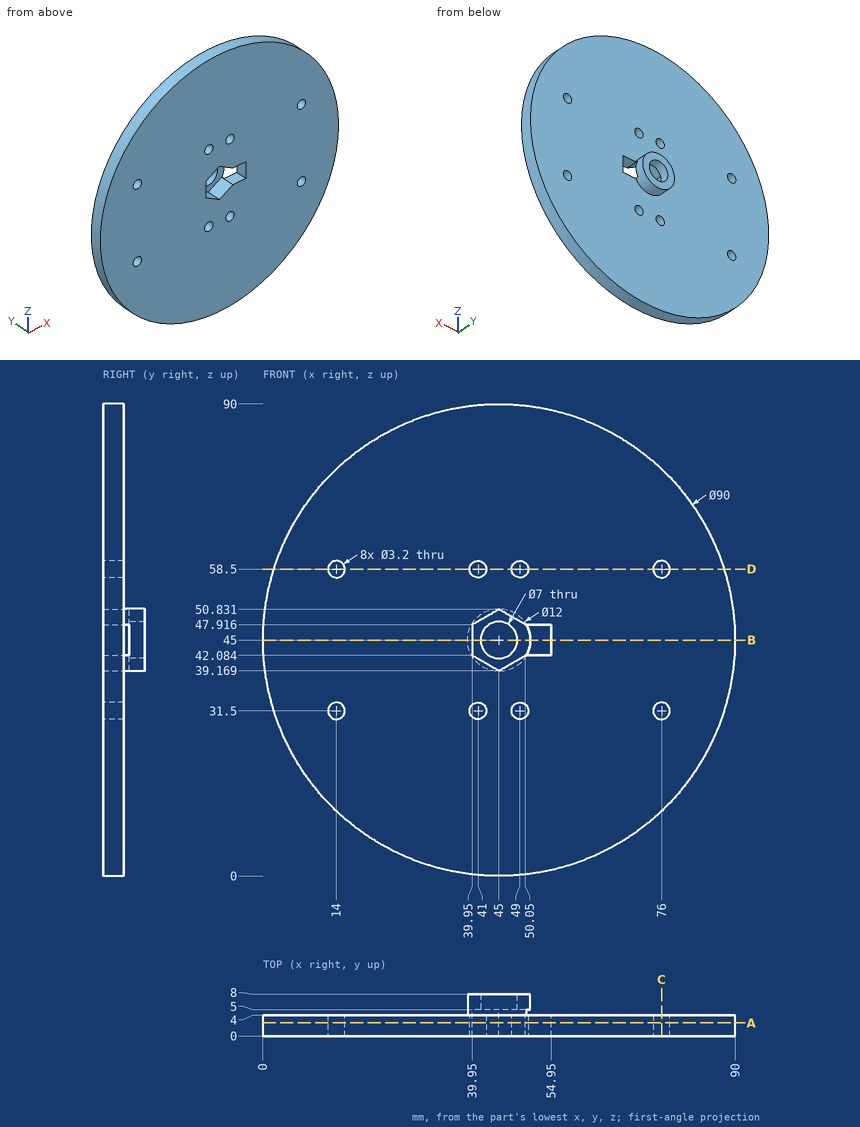
Geometry check sheet. Reference: drawing and pictorial views, mm from the part's lowest x, y, z. Round coordinates to 2 decimals unless told otherwise and drop trailing zeros. Order: outer loops, then holes, each group sorted by start corner. A loop starts at its lowest first (then second) coordinate and runs counter-clockwise, first axis right, second up. Notation, with made-up numbers: M -35.5,-8 L 6.5,-8 A28 ccw 6.5,10 Z; hole C 85.5,85 d6. An arc over 180 degrees is marked long. Answer in a Markdown table with one row per item.
(1) Scan lines: probe 1 along Z at (x, y) = (14, 1.9); probe 2 along Z at (x, y) = (49, 2.75); probe 3 along Y at (x, z) = (20, 13). Record each from-to range of solid material in increasing order. Write a range as from..to.
Responses:
| item | result |
|---|---|
| probe 1 | z = 12.38..29.9, 33.1..56.9, 60.1..77.62 |
| probe 2 | z = 0.18..29.9, 33.1..41.48, 48.52..56.9, 60.1..89.82 |
| probe 3 | y = 0..4 |
(2) Sectioned sample at C-C, the plane x = 76. Record the cut outline in (y, z), and give its area (3 significant figures).
Responses:
| item | result |
|---|---|
| outline | M 0,12.38 L 4,12.38 L 4,29.9 L 0,29.9 Z; M 0,33.1 L 4,33.1 L 4,56.9 L 0,56.9 Z; M 0,60.1 L 4,60.1 L 4,77.62 L 0,77.62 Z |
| area | 235 mm² |
(3) Sectioned sample at A-A, the plane y = 2.5. State how many separate pieces and enclosed holes the cut face has, and give its area (3 significant figures).
Responses:
| item | result |
|---|---|
| separate pieces | 1 |
| enclosed holes | 9 |
| area | 6,180 mm² |
(4) Go/stop test with flat-tipped pins: P1, Ø3, axis at x = 49, z = 58.5, coming from the -Y side; P2, Ø2.5, axis at y = 1.5, z = 43.5, coming from the +X side; P3, Ø3.5, axis at x = 76, z = 58.5, coming from the +Y side; P4, Ø2.5, axis at x = 53, y = 1.5, coming from the +Z side. Record where each tip stops, or that it passes through.
Responses:
| item | result |
|---|---|
| P1 | passes through |
| P2 | stops at x = 90 |
| P3 | stops at y = 4 |
| P4 | stops at z = 89.49 |
(5) Sectioned sample at B-B, the plane z = 45. Record the cut outline in (x, y), and give its area (3 significant figures).
Responses:
| item | result |
|---|---|
| outline | M 0,0 L 39.95,0 L 39.95,5 L 41.5,5 L 41.5,8 L 39,8 L 39,4 L 0,4 Z; M 48.5,5 L 51,5 L 51,8 L 48.5,8 Z; M 54.95,0 L 90,0 L 90,4 L 54.95,4 Z |
| area | 316 mm² |
(6) Sectioned sample at D-D, the plane z = 58.5. Record the cut outline in (x, y), and give its area (3 significant figures).
Responses:
| item | result |
|---|---|
| outline | M 2.07,0 L 12.4,0 L 12.4,4 L 2.07,4 Z; M 15.6,0 L 39.4,0 L 39.4,4 L 15.6,4 Z; M 42.6,0 L 47.4,0 L 47.4,4 L 42.6,4 Z; M 50.6,0 L 74.4,0 L 74.4,4 L 50.6,4 Z; M 77.6,0 L 87.93,0 L 87.93,4 L 77.6,4 Z |
| area | 292 mm² |
